from build123d import *

# Parameters (mm, degrees)
BOSS_EXTRUDE1_DEPTH = 30
BOSS_EXTRUDE2_START = -20
BOSS_EXTRUDE2_DEPTH = 20


# Read off the part's stored shape, not the designer's step: Boss-Extrude2
with BuildPart() as part:
    # Sketch1 → Boss-Extrude1 (new body)
    with BuildSketch(Plane(origin=(0, 0, 0), x_dir=(1, 0, 0), z_dir=(0, 1, 0))):
        with BuildLine():
            Line((0, 80), (300, 80))
            ThreePointArc((300, 80), (380, 0), (300, -80))
            Line((300, -80), (0, -80))
            ThreePointArc((0, -80), (-80, 0), (0, 80))
        make_face()
    extrude(amount=BOSS_EXTRUDE1_DEPTH)

    # Boss-Extrude2 outline → Boss-Extrude2 (cut)
    with BuildSketch(Plane(origin=(0, 30, 0), x_dir=(1, 0, 0), z_dir=(0, 1, 0)).offset(BOSS_EXTRUDE2_START)):
        with BuildLine():
            Line((0, -70), (300, -70))
            ThreePointArc((300, -70), (370, 0), (300, 70))
            Line((300, 70), (0, 70))
            ThreePointArc((0, 70), (-70, 0), (0, -70))
        make_face()
    extrude(amount=BOSS_EXTRUDE2_DEPTH, mode=Mode.SUBTRACT)


solid = part.part
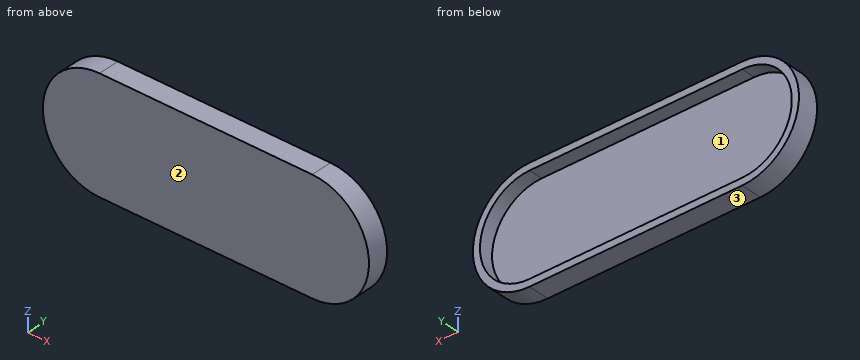
Verification items for the finished model (mm, model axes). Face numbers are marked on the shaded views. Coordinates: 2 decimals unless noted, no trailing zeros. Loops run counter-clockwise (first coordinate to the right, second up) from the corner with the lowest first, then second, coordinate; pieces in that order, holes last. Notation, with made-up numbers: (87.5, 71) -> (115.5, 71) arc R15 cw to (115.5, 94) -> close; hole circle Ø11 at (84, 50). An arc over 180 degrees is marked (long way). Answer as CSV lines item,"result".
1) Cross-section at A-A, the plane y = 14.5. Record the cut outline in (x, z).
Found:
outline,"(0, -80) -> (300, -80) arc R80 ccw to (300, 80) -> (0, 80) arc R80 ccw to start; hole (0, -70) -> (300, -70) arc R70 ccw to (300, 70) -> (0, 70) arc R70 ccw to start"
2) Cross-section at C-C, the plane z = 0. Record the cut outline in (x, y), then the cut area to 3 significant figures.
Found:
outline,"(-80, 0) -> (380, 0) -> (380, 30) -> (370, 30) -> (370, 10) -> (-70, 10) -> (-70, 30) -> (-80, 30) -> close"
area,"5,000 mm2"
3) Release check for a two-part mould opening along Z. For the marked faces 1, 2 and 3 record: +Z half, -Z half, draft (parallel to the pull), parting line (faces both ways), or undercut.
Found:
face 1,"undercut"
face 2,"draft"
face 3,"-Z half"
4) Depth check by flat-ended pin: pin 1 (12 mm diameter, centred on y = 12.5, z = -34, fed in from +X); pin 2 (10 mm diameter, centred on y = 10.5, z = 19, fed in from -X); pin 3 (3 mm diameter, centred on y = 17.5, z = 55.5, fed in from +X). Enter the tip coordinate at first touch or a pass-through.
Found:
pin 1,"stops at x = 374.94"
pin 2,"stops at x = -78.77"
pin 3,"stops at x = 359.03"
5) Cross-section at B-B, the plane x = 289. Record the cut outline in (y, z).
Found:
outline,"(0, -80) -> (30, -80) -> (30, -70) -> (10, -70) -> (10, 70) -> (30, 70) -> (30, 80) -> (0, 80) -> close"
6) Thickness scan on L1, parallel to Z at x = 0.5, y = 15; L2, parallel to X at y = 21, z = -3.5; L3, parallel to Y at x = 207, z = 43. Record the ranges inside material, lowest first. Write a range as from..to.
Found:
L1,"z = -80..-70, 70..80"
L2,"x = -79.92..-69.91, 369.91..379.92"
L3,"y = 0..10"
